from build123d import *

# Parameters (mm, degrees)
F0_R     = 11
F0_R_2   = 7.5
F1_DEPTH = 2
F0_R_3   = 4.275
F2_DEPTH = 3
F3_DEPTH = 1.7
F4_R     = 0.99999


# Not quite as in the source:
# - a fillet or chamfer is up to 0.001 mm smaller than in the source, because OpenCascade refuses the exact size


with BuildPart() as f1:
    # F0 (on Top) → F1 (new body)
    with BuildSketch(Plane.XY):
        Circle(F0_R)
        Circle(F0_R_2, mode=Mode.SUBTRACT)
    extrude(amount=F1_DEPTH)

    # F0 (on Top) → F2 (join)
    with BuildSketch(Plane.XY):
        Circle(F0_R_2)
        Circle(F0_R_3, mode=Mode.SUBTRACT)
    extrude(amount=F2_DEPTH)

    # F0 (on Top) → F3 (join)
    with BuildSketch(Plane.XY):
        Circle(F0_R_3)
    extrude(amount=F3_DEPTH)

    # F4 (radius 1 in the source; OpenCascade refuses exactly that, so slightly less here)
    f4_edges = [f1.edges().sort_by_distance(p)[0] for p in [
        (-11, 0, 2),
        (-11, 0, 0),
    ]]
    fillet(f4_edges, radius=F4_R)


solid = f1.part
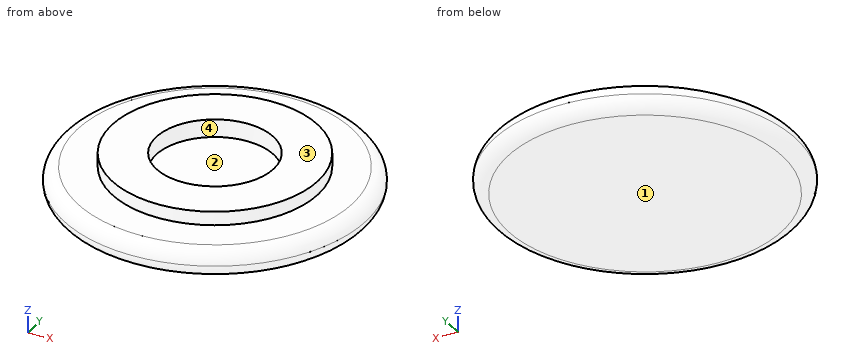
Can you work these out from the model? Positions are in its coordinate system, mm. Face numbers are marked on the shaded views. A direction names the side the tool comes from. Round coordinates to 2 decimals unless told otherwise and drop trailing zeros. Write each loop counter-clockwise with the first axis right and the second up, starting at its lowest first coordinate (ties: lowest second). Pieces come first, ordered by that corner, then holes. Notation, with made-up numbers: (86, 76) -> (104, 76) arc R26 cw to (104, 95) -> close; hole circle Ø11 at (57, 82.5). An arc over 180 degrees is marked (long way). One line per question, with ' | ' between items. Start each with the question number.
1) Suppose I cut it at C-C on z = 0.4. Write out the boundary of the cut face in (x, y), then the cut area to 3 significant figures.
2) If we mould it in two halves opening along X, with no side actions, what happens to the marked faces 1 and 2? For each: released by +X, released by -X, zero draft, split by the parting line, or undercut.
3) On a 3-axis mill with a long thin cutter (end or side, diameter ignored), from which of +Z, -Z, +X, -X, +Y, -Y can I reach the whole of each face in a straight line? I mean the marked faces 3 and 4. Say none if no direction works.
4) I'm going to push flat-ended pins straight in: P1, Ø1, axis at x = 1.5, z = 2, coming from the +Y side; P2, Ø2.5, axis at x = 0, y = 0.5, coming from the +Z side; P3, Ø2, axis at x = -8, y = -8, coming from the +Z side. Where does each tip first touch, or does it pass through?
5) I need wall thicknesses on line 1 (Y direction, x = 0, z = 2.3) (3 decimals); line 2 (Y direction, x = 0.5, z = 2.5); line 3 (Z direction, x = 5.75, y = 8). Which ranges of each line are inside material? Lowest first, please. Write a range as [from, to].
Return value:
1) outline: circle Ø21.6 at (0, 0) | area: 366 mm2
2) face 1: zero draft | face 2: undercut
3) face 3: +Z, +X, -X, +Y, -Y | face 4: +Z
4) P1: stops at y = 10.77 | P2: stops at z = 1.7 | P3: stops at z = 1.95
5) line 1: y = [-7.5, -4.275], [4.275, 7.5] | line 2: y = [-7.48, -4.25], [4.25, 7.48] | line 3: z = [0, 2]
